Source: CAD feature listing. Evaluate the final solid. Frame: model axes, mm. A direction names the side the tool comes from. Round coordinates to 2 decimals unless told otherwise and drop trailing zeros. Loops run counter-clockwise (first coordinate to the right, second up) from the corner with the lowest first, then second, coordinate; pieces in that order, holes last. Notation, with made-up numbers: (75.5, -8.5) -> (116.5, -8.5) arc R20 cw to (116.5, -0.5) -> close; hole circle Ø2 at (30.25, 0). An arc over 180 degrees is marked (long way). Write item = value, one per line.
from build123d import *

# Parameters (mm, degrees)
IZIM1_W                   = 505
IZIM1_H                   = 150
TABAN_FLAN_1_DEPTH        = 10
IZIM6_R                   = 4.25
KES_EKSTR_ZYON1_DEPTH     = 264.592962729
AYNALAMA2_COPY_1_SKETCH_R = 4.25
AYNALAMA2_COPY_1_DEPTH    = 264.592962729
IZIM7_W                   = 22.5
IZIM7_H                   = 43
IZIM7_W_2                 = 177.5
SEKME1_DEPTH              = 10


# Sheet-metal steps are written as plain solids
with BuildPart() as part:
    # Çizim1 → Taban-Flanş1 (new body)
    with BuildSketch(Plane.XY):
        Rectangle(IZIM1_W, IZIM1_H)
    extrude(amount=-TABAN_FLAN_1_DEPTH)

    # Çizim6 → Kes-Ekstrüzyon1 (cut, through all)
    with BuildSketch(Plane(origin=(0, 0, -10), x_dir=(-1, 0, 0), z_dir=(0, 0, -1))):
        with Locations((245, -67.5)):
            Circle(IZIM6_R)
    kes_ekstr_zyon1 = extrude(amount=-KES_EKSTR_ZYON1_DEPTH, mode=Mode.SUBTRACT)

    # Aynalama1: Kes-Ekstrüzyon1 across plane
    add(kes_ekstr_zyon1.mirror(Plane(origin=(0, 0, 0), x_dir=(0, 0, 1), z_dir=(1, 0, 0))), mode=Mode.SUBTRACT)

    # Aynalama2: Kes-Ekstrüzyon1 across plane
    add(kes_ekstr_zyon1.mirror(Plane.ZX), mode=Mode.SUBTRACT)

    # Aynalama2 copy 1 sketch → Aynalama2 copy 1 (cut, through all)
    with BuildSketch(Plane(origin=(0, 0, -10), x_dir=(1, 0, 0), z_dir=(0, 0, -1))):
        with Locations((245, -67.5)):
            Circle(AYNALAMA2_COPY_1_SKETCH_R)
    extrude(amount=-AYNALAMA2_COPY_1_DEPTH, mode=Mode.SUBTRACT)

    # Çizim7 → Sekme1 (add)
    with BuildSketch(Plane.XY):
        with Locations((-241.25, -96.5)):
            Rectangle(IZIM7_W, IZIM7_H)
        with Locations((-106.25, -96.5)):
            Rectangle(IZIM7_W_2, IZIM7_H)
        with Locations((106.25, -96.5)):
            Rectangle(IZIM7_W_2, IZIM7_H)
        with Locations((241.25, -96.5)):
            Rectangle(IZIM7_W, IZIM7_H)
    extrude(amount=-SEKME1_DEPTH)


solid = part.part
1. Section query A-A (z = -6.25). Return the cut outline in (x, y), then the cut area to 3 significant figures.
Evaluation:
outline = (-252.5, -118) -> (-230, -118) -> (-230, -75) -> (-195, -75) -> (-195, -118) -> (-17.5, -118) -> (-17.5, -75) -> (17.5, -75) -> (17.5, -118) -> (195, -118) -> (195, -75) -> (230, -75) -> (230, -118) -> (252.5, -118) -> (252.5, 75) -> (-252.5, 75) -> close; hole circle Ø8.5 at (-245, -67.5); hole circle Ø8.5 at (-245, 67.5); hole circle Ø8.5 at (245, -67.5); hole circle Ø8.5 at (245, 67.5)
area = 92,700 mm²
2. Set-up query: faces 5 (the face through (230, -97, -5)), 6 (the face through (-4, -20, 0)). Return all of +Z, -Z, +X, -X, +Y, -Y with unobstructed straight access to the full face (end or side cutting, diameter ignored); none if empty.
Evaluation:
face_5 = +Z, -Z, -Y
face_6 = +Z, +X, -X, +Y, -Y
3. Section query B-B (x = 4.5). Return the cut outline in (y, z).
Evaluation:
outline = (-75, -10) -> (75, -10) -> (75, 0) -> (-75, 0) -> close
4. Contact query for flat-ended pins moving along their axis: pin 1 Ø3 at (x, z) = (-212.5, -4.5) entering from -Y; pin 2 Ø7 at (x, y) = (245, -67.5) entering from -Z. Output: stop coordinate, or through.
Evaluation:
pin_1 = -75
pin_2 = through
5. Line query: probe 1 along Y at (x, z) = (245, -3); probe 2 along X at (y, z) = (67.5, -5.5); probe 3 along X at (y, z) = (-92, -1.5). Output: solid intervals per line, ascending. Write a range as from..to.
Evaluation:
probe_1 = -118..-71.75, -63.25..63.25, 71.75..75
probe_2 = -252.5..-249.25, -240.75..240.75, 249.25..252.5
probe_3 = -252.5..-230, -195..-17.5, 17.5..195, 230..252.5
6. Mould query, pull axis Y, two halves, no side actions, for faces 1 (the face through (-4, 75, -5)), 2 (the face through (-195, -97, -5)), 3 (the face through (240.754, 67.313, -5.07)), 4 (the face through (-213, -75, -5)). Classes: released by +Y, released by -Y, zero draft, split by the parting line, or undercut.
Evaluation:
face_1 = released by +Y
face_2 = zero draft
face_3 = undercut
face_4 = released by -Y
